Source: CAD feature listing. Evaluate the final solid. Frame: model axes, mm. Face numbers are marked on the shaded views. A direction names the side the tool comes from. Give positions to 0.01 mm unless a question says otherwise; leave off trailing zeros. Loops run counter-clockwise (first coordinate to the right, second up) from the corner with the lowest first, then second, coordinate; pieces in that order, holes last. Notation, with made-up numbers: M -40,40.5 L -20,40.5 A27 cw -20,68.5 Z; hole C 11,29 d2. An arc over 180 degrees is marked long. Answer in a Markdown table with one row per item.
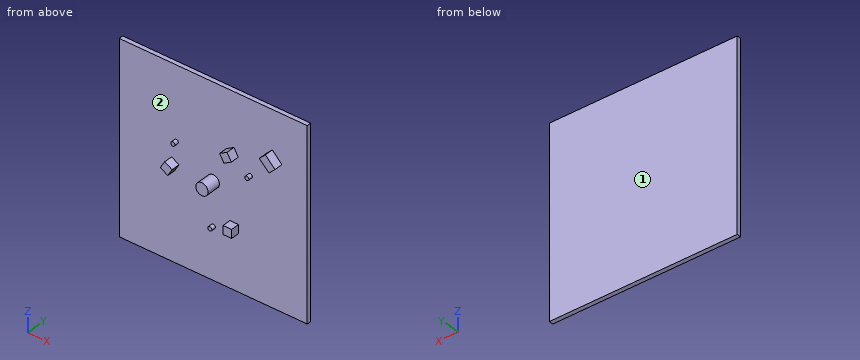
```python
from build123d import *

# Parameters (mm, degrees)
F0_W      = 1100
F0_H      = 1100
F1_DEPTH  = 25
F2_R      = 36.0100678946
F3_DEPTH  = 82
F4_R      = 12
F5_DEPTH  = 25
F6_DEPTH  = 25
F7_W      = 50
F7_H      = 50
F8_DEPTH  = 50
F10_DEPTH = 50


# Not quite as in the source:
# - a feature names something its author has since deleted; it is built from what else it names


with BuildPart() as f1:
    # F0 (on Front) → F1 (new body)
    with BuildSketch(Plane.XZ):
        Rectangle(F0_W, F0_H)
    extrude(amount=F1_DEPTH)

    # F2 (on face) → F3 (join)
    with BuildSketch(Plane.XZ.offset(25)):
        Circle(F2_R)
    extrude(amount=F3_DEPTH)

    # F4 (on face) → F5 (join)
    with BuildSketch(Plane.XZ.offset(25)):
        with Locations((0, -250)):
            Circle(F4_R)
    extrude(amount=F5_DEPTH)

    # F4 (on face) → F6 (join)
    with BuildSketch(Plane.XZ.offset(25)):
        with Locations((-216.5063509461, 125)):
            Circle(F4_R)
        with Locations((216.5063509461, 125)):
            Circle(F4_R)
    extrude(amount=F6_DEPTH)

    # F7 (on face) → F8 (join)
    with BuildSketch(Plane.XZ.offset(25)):
        Polygon((121.1628514659, 240.6145112228), (77.8615812767, 215.6145112228), (102.8615812767, 172.3132410336), (146.1628514659, 197.3132410336), align=None)
        with Locations((122.7968535052, -200.2373629758)):
            Rectangle(F7_W, F7_H)
        Polygon((-268.9597049711, -15.377148247), (-225.6584347818, -40.377148247), (-200.6584347818, 2.9241219422), (-243.9597049711, 27.9241219422), align=None)
    extrude(amount=F8_DEPTH)

    # F9 (on face) → F10 (join)
    with BuildSketch(Plane.XZ.offset(25)):
        Polygon((345.3553390593, 325.3553390593), (310, 290), (366.5685424949, 233.4314575051), (401.9238815543, 268.7867965644), align=None)
    extrude(amount=F10_DEPTH)


solid = f1.part
```
Q1. Contact query for flat-ended pins moving along their axis: pin 1 Ø7 at (x, z) = (-221.5, 127.5) entering from -Y; pin 2 Ø8 at (x, y) = (94.5, -65.5) entering from +Z; pin 3 Ø3 at (x, z) = (-120.5, -78) entering from -Y; pin 4 Ø5 at (x, z) = (412, 30) entering from +Y. Output: stop coordinate, or through.
Values follow:
| item | result |
|---|---|
| pin 1 | y = -50 |
| pin 2 | z = 227.53 |
| pin 3 | y = -25 |
| pin 4 | y = 0 |
Q2. Ray query, probe 1 along Y at (x, z) = (377.5, 207); probe 2 along X at (y, z) = (-43, -206); probe 3 along X at (y, z) = (-48, 178). Return the intervals inside material, ascending. Write a range as from..to.
Values follow:
| item | result |
|---|---|
| probe 1 | -25..0 |
| probe 2 | 97.8..147.8 |
| probe 3 | 99.58..112.71 |
Q3. Section query D-D (z = -401.5). Output: boundary loops of the cut face in (x, y).
Values follow:
| item | result |
|---|---|
| outline | M -550,-25 L 550,-25 L 550,0 L -550,0 Z |
Q4. Section query A-A (z = -195.5). Output: boundary loops of the cut face in (x, y), plus the area to 3 significant figures.
Values follow:
| item | result |
|---|---|
| outline | M -550,-25 L 97.8,-25 L 97.8,-75 L 147.8,-75 L 147.8,-25 L 550,-25 L 550,0 L -550,0 Z |
| area | 30,000 mm^2 |
Q5. Section query B-B (y = -92.5). Output: boundary loops of the cut face in (x, z).
Values follow:
| item | result |
|---|---|
| outline | C 0,0 d72.02 |
Q6. Section query C-C (x = -474.5). Output: boundary loops of the cut face in (y, z).
Values follow:
| item | result |
|---|---|
| outline | M -25,-550 L 0,-550 L 0,550 L -25,550 Z |
Q7. Reachability of the marked faces 1 and 2 from +Z, -Z, +X, -X, +Y, -Y: full face, straight path, thin tool, end or side. Return the list, or none.
Values follow:
| item | result |
|---|---|
| face 1 | +Z, -Z, +X, -X, +Y |
| face 2 | -Y |
